Answer from the drawing. Dimensions are ordinates in mm from the lowest x, y and z of the part. A direction names the side the tool comes from. Give positions to 0.01 mm unless a question says otherwise; leave off trailing zeros. Write each loop counter-clockwise with the first axis right and the second up, starting at its lowest first coordinate (ties: lowest second). Pieces come first, ordered by that corner, then holes.
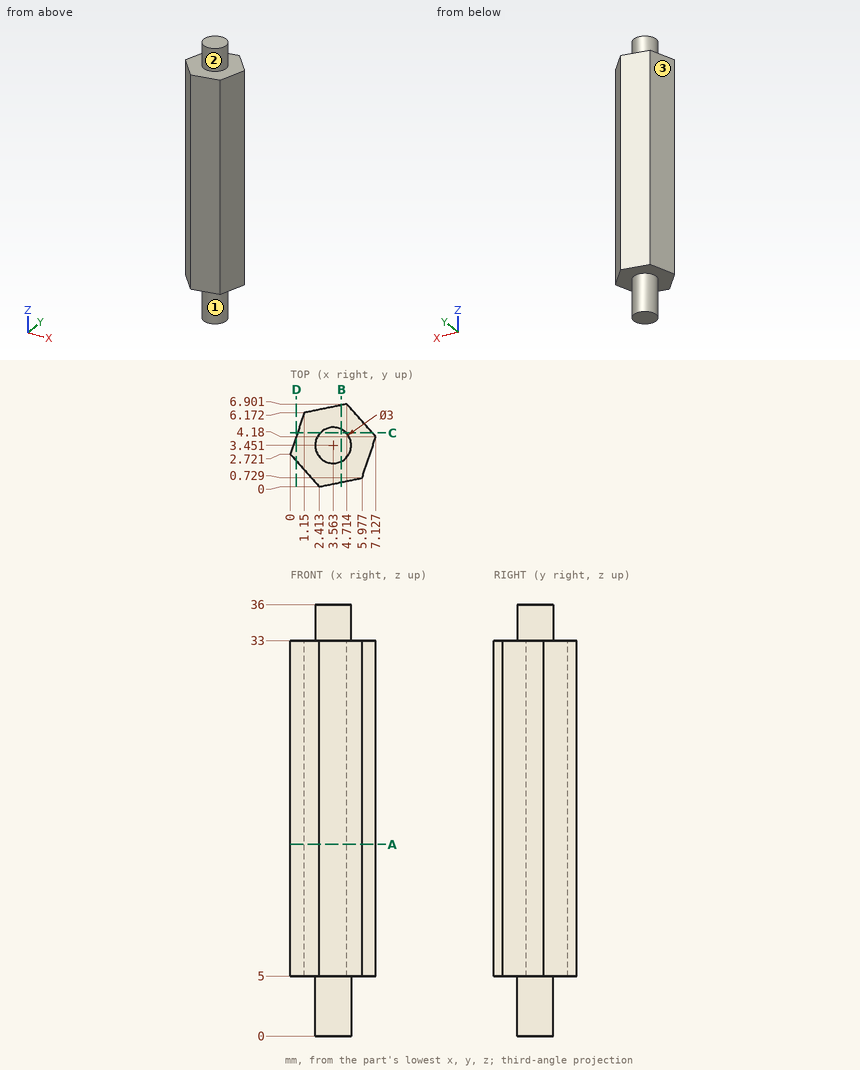
Item 1: Which of the six approach directions +Z, -Z, +X, -X, +Y, -Y give full straight-line access (tool end or side, diameter ignored) to the marked faces 1, 2 and 3?
Conclusion:
face 1: -Z
face 2: +Z
face 3: +Z, -Z, -X, +Y
Item 2: A cutting plane is placed at A-A, the plane z = 16. Give the vertices of the cut face in (x, y), plus the area to 3 significant figures.
Conclusion:
outline: (0, 2.72) - (2.41, 0) - (5.98, 0.73) - (7.13, 4.18) - (4.71, 6.9) - (1.15, 6.17) - close
area: 34.4 mm2
Item 3: A cutting plane is placed at D-D, the plane x = 0.5. Give the vertices of the cut face in (y, z).
Conclusion:
outline: (2.16, 5) - (4.22, 5) - (4.22, 33) - (2.16, 33) - close
Item 4: Each of these flat-tipped pins is pushed along its axis until it touches: P1, Ø1, axis at x = 1, y = 5.5, coming from the +Z side; P2, Ø3, axis at y = 1.5, z = 23, coming from the +X side; P3, Ø1, axis at y = 6, z = 15.5, coming from the -X side. Where does it stop, or does it pass through?
Conclusion:
P1: stops at z = 33
P2: stops at x = 6.73
P3: stops at x = 0.93
Item 5: Consider probe 1 along Z at (x, y) = (3.75, 1.5); probe 2 along Y at (x, z) = (4.25, 8.5) (1 decimal); probe 3 along X at (y, z) = (3, 5.5) (1 decimal). Determine where each line is inside the solid, lowest interval first.
Conclusion:
probe 1: z = 5 to 33
probe 2: y = 0.4 to 6.8
probe 3: x = 0.1 to 6.7
Item 6: A cutting plane is placed at C-C, the plane y = 4.5. Give the vertices of the cut face in (x, z) (1 decimal).
Conclusion:
outline: (0.6, 5) - (2.5, 5) - (2.5, 0) - (4.6, 0) - (4.6, 5) - (6.8, 5) - (6.8, 33) - (4.6, 33) - (4.6, 36) - (2.5, 36) - (2.5, 33) - (0.6, 33) - close
Item 7: A cutting plane is placed at B-B, the plane x = 4.25. Give the vertices of the cut face in (y, z) (1 decimal).
Conclusion:
outline: (0.4, 5) - (2.1, 5) - (2.1, 0) - (4.8, 0) - (4.8, 5) - (6.8, 5) - (6.8, 33) - (4.8, 33) - (4.8, 36) - (2.1, 36) - (2.1, 33) - (0.4, 33) - close
